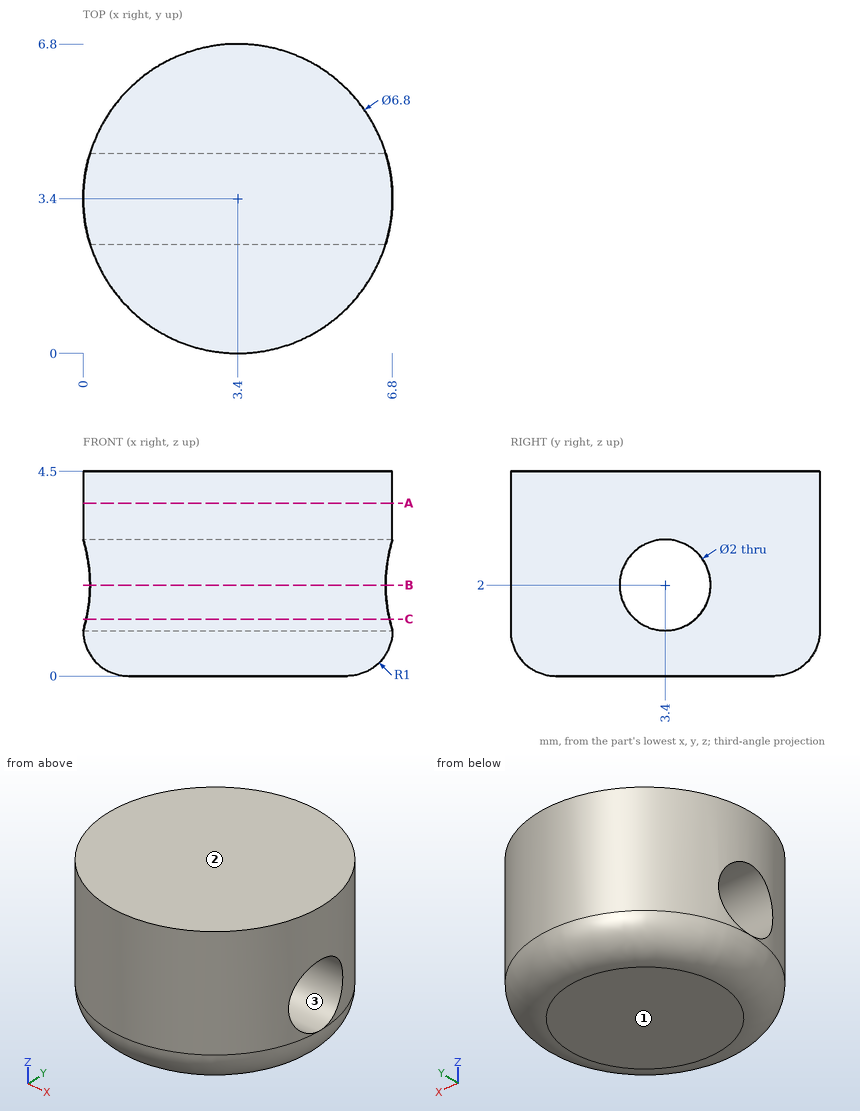
Source: three-view drawing plus pictorial views. Frame: mm from the lowest corner of the part. Round coordinates to 2 decimals unless told otherwise and drop trailing zeros. Loops run counter-clockwise (first coordinate to the right, second up) from the corner with the lowest first, then second, coordinate; pieces in that order, holes last.
Q1. Ray query, line 1 (Y direction, x = 4.5, z = 2); line 2 (Y direction, x = 5.5, z = 2); line 3 (Y direction, x = 4.25, z = 3.55). Return the intervals inside material, ascending.
Q2. Section B-B, the plane z = 2. Return loops of the section in (x, y).
Q3. Section A-A, the plane z = 3.8. Return loops of the section in (x, y), plus the area to 3 significant figures.
Q4. Section C-C, the plane z = 1.25. Return loops of the section in (x, y) (1 decimal), plus the area to 3 significant figures.
Q5. Mould query, pull axis Z, two halves, no side actions, for the marked faces 1, 2 and 3. Classes: pulls with the +Z half, pulls with the -Z half, needs draft (parallel to the pull), parting line crosses it, or undercut.
Solutions:
1. line 1: y = 0.18 to 2.4, 4.4 to 6.62
1. line 2: y = 0.73 to 2.4, 4.4 to 6.07
1. line 3: y = 0.11 to 6.69
2. outline: (0.15, 2.4) arc R3.4 ccw to (6.65, 2.4) - close; (0.15, 4.4) - (6.65, 4.4) arc R3.4 ccw to start
3. outline: circle Ø6.8 at (3.4, 3.4)
3. area: 36.3 mm2
4. outline: (0.1, 2.7) arc R3.4 ccw to (6.7, 2.7) - close; (0.1, 4.1) - (6.7, 4.1) arc R3.4 ccw to start
4. area: 27.4 mm2
5. face 1: pulls with the -Z half
5. face 2: pulls with the +Z half
5. face 3: undercut
